Geometry: see drawing. Coordinates: mm, zero at the bounding-box minimum. Coordinates: 2 decimals unless noted, no trailing zeros. Write each loop counter-clockwise with the first axis right and the second up, starting at its lowest first coordinate (ties: lowest second). Pieces come first, ordered by that corner, then holes.
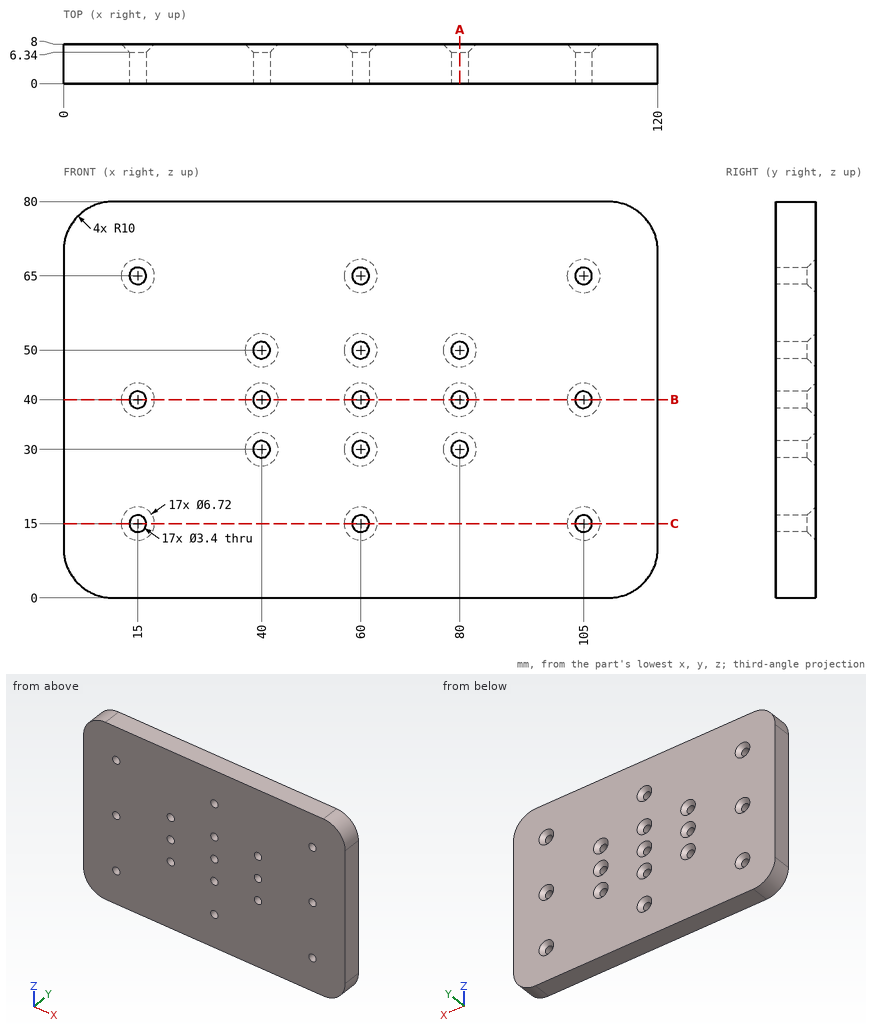
Item 1: Material intervals for probe 1 along X at (y, z) = (2.75, 40); probe 2 along Z at (x, y) = (40, 2); probe 3 along Z at (x, y) = (15, 5), sorted ascending.
Derived:
probe 1: x = 0 to 13.3, 16.7 to 38.3, 41.7 to 58.3, 61.7 to 78.3, 81.7 to 103.3, 106.7 to 120
probe 2: z = 0 to 28.3, 31.7 to 38.3, 41.7 to 48.3, 51.7 to 80
probe 3: z = 0 to 13.3, 16.7 to 38.3, 41.7 to 63.3, 66.7 to 80
Item 2: Section B-B, the plane z = 40. State how many separate pieces and enclosed holes the cut face has, plus the area to 3 significant figures.
Derived:
separate pieces: 6
enclosed holes: 0
area: 810 mm2
Item 3: Section C-C, the plane z = 15. Output: boundary loops of the cut face in (x, y).
Derived:
outline: (0, 0) - (13.3, 0) - (13.3, 6.34) - (11.64, 8) - (0, 8) - close; (16.7, 0) - (58.3, 0) - (58.3, 6.34) - (56.64, 8) - (18.36, 8) - (16.7, 6.34) - close; (61.7, 0) - (103.3, 0) - (103.3, 6.34) - (101.64, 8) - (63.36, 8) - (61.7, 6.34) - close; (106.7, 0) - (120, 0) - (120, 8) - (108.36, 8) - (106.7, 6.34) - close
Item 4: Section A-A, the plane x = 80. Output: boundary loops of the cut face in (y, z), plus the area to 3 significant figures.
Derived:
outline: (0, 0) - (8, 0) - (8, 26.64) - (6.34, 28.3) - (0, 28.3) - close; (0, 31.7) - (6.34, 31.7) - (8, 33.36) - (8, 36.64) - (6.34, 38.3) - (0, 38.3) - close; (0, 41.7) - (6.34, 41.7) - (8, 43.36) - (8, 46.64) - (6.34, 48.3) - (0, 48.3) - close; (0, 51.7) - (6.34, 51.7) - (8, 53.36) - (8, 80) - (0, 80) - close
area: 550 mm2
Item 5: Pin query (flat end, axial travel): pin 1 (3 mm diameter, centred on x = 15, z = 65, fed in from +Y); pin 2 (4 mm diameter, centred on x = 60, z = 65, fed in from +Y); pin 3 (5.5 mm diameter, centred on x = 60, z = 30, fed in from +Y). Return the tip coordinate at first contact, or that it passes through.
Derived:
pin 1: passes through
pin 2: stops at y = 6.64
pin 3: stops at y = 7.39
